Check sheet for the drawn part. Datum: minimum x, y, z corner. Units: mm. A direction names the side the tool comes from. Round coordinates to 2 decimals unless told otherwise and drop trailing zeros. Order: outer loops, then holes, each group sorted by start corner. A loop starts at its lowest first (then second) coordinate and runs counter-clockwise, first axis right, second up. Notation, with made-up numbers: M -23,66 L -6,66 A32 ccw -6,93 Z; hole C 5,-39 d10. An arc over 180 degrees is marked long. Use one line per item in the form item = value. Start each with the question number.
Item 1: Cross-section at D-D on z = 444. Enter the section's corners in (x, y).
Item 2: Tool access check on the marked faces 1, 2 and 3. Record the directions out of +Z, -Z, +X, -X, +Y, -Y that give a thin tool (end or side, any length) a straight path to the whole face; none if there is none.
Item 3: Go/stop test with flat-tipped pins: pin 1 Ø8 at (x, y) = (40, 74) entering from -Z; pin 2 Ø1 at (x, z) = (65, 203) entering from -Y; pin 3 Ø1.5 at (x, z) = (39, 142.5) entering from +Y. Record where each tip stops, or that it passes through.
Item 4: Cross-section at C-C on z = 236. Enter the section's corners in (x, y).
Item 5: Thickness scan on probe 1 along Z at (x, y) = (62, 89); probe 2 along X at (y, z) = (75.5, 277); probe 3 along Y at (x, z) = (60.5, 197). Record the ranges inside material, lowest first. Write a range as [from, to].
Item 6: Cross-section at A-A on y = 50.8. Enter the section's corners in (x, z).
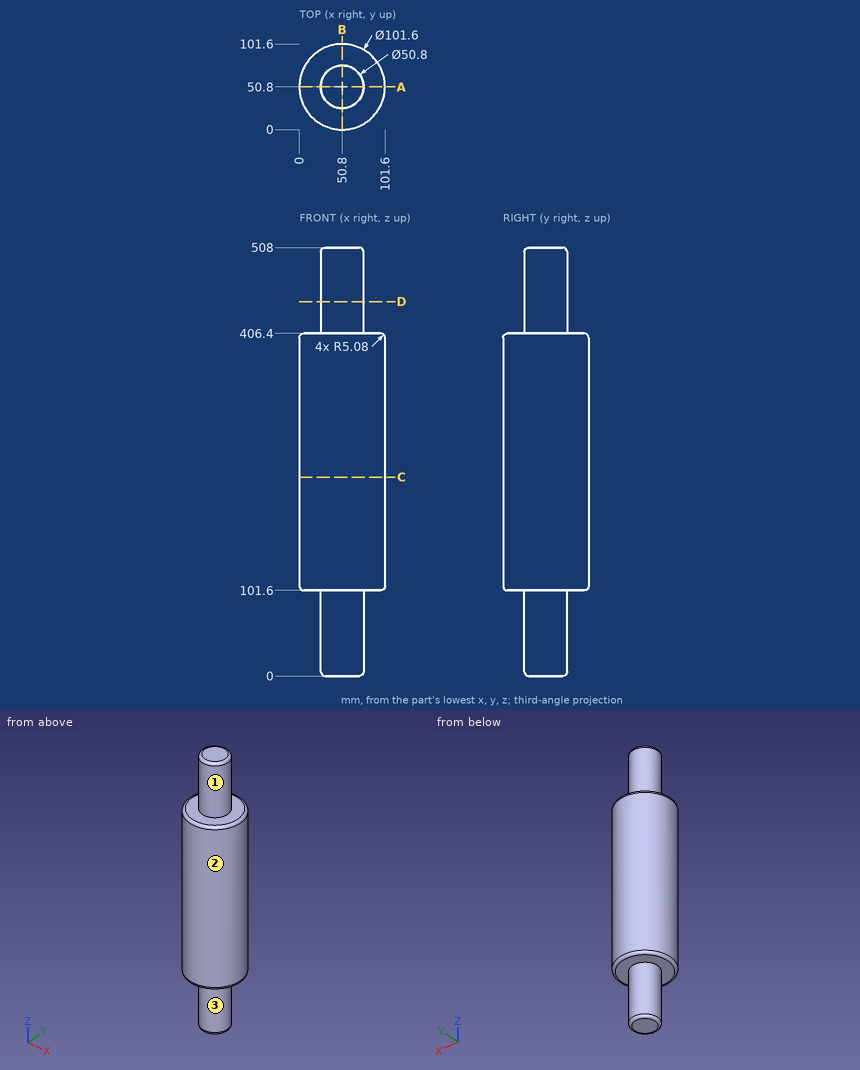
Output values:
q1.outline = C 50.8,50.8 d50.8
q2.face_1 = +Z
q2.face_2 = +Z, -Z
q2.face_3 = -Z
q3.pin_1 = 0.16
q3.pin_2 = 1.88
q3.pin_3 = 100.38
q4.outline = C 50.8,50.8 d101.6
q5.probe_1 = [101.6, 406.4]
q5.probe_2 = [6.41, 95.19]
q5.probe_3 = [0.93, 100.67]
q6.outline = M 0,106.68 A5.08 ccw 5.08,101.6 L 25.4,101.6 L 25.4,5.08 A5.08 ccw 30.48,0 L 71.12,0 A5.08 ccw 76.2,5.08 L 76.2,101.6 L 96.52,101.6 A5.08 ccw 101.6,106.68 L 101.6,401.32 A5.08 ccw 96.52,406.4 L 76.2,406.4 L 76.2,502.92 A5.08 ccw 71.12,508 L 30.48,508 A5.08 ccw 25.4,502.92 L 25.4,406.4 L 5.08,406.4 A5.08 ccw 0,401.32 Z
